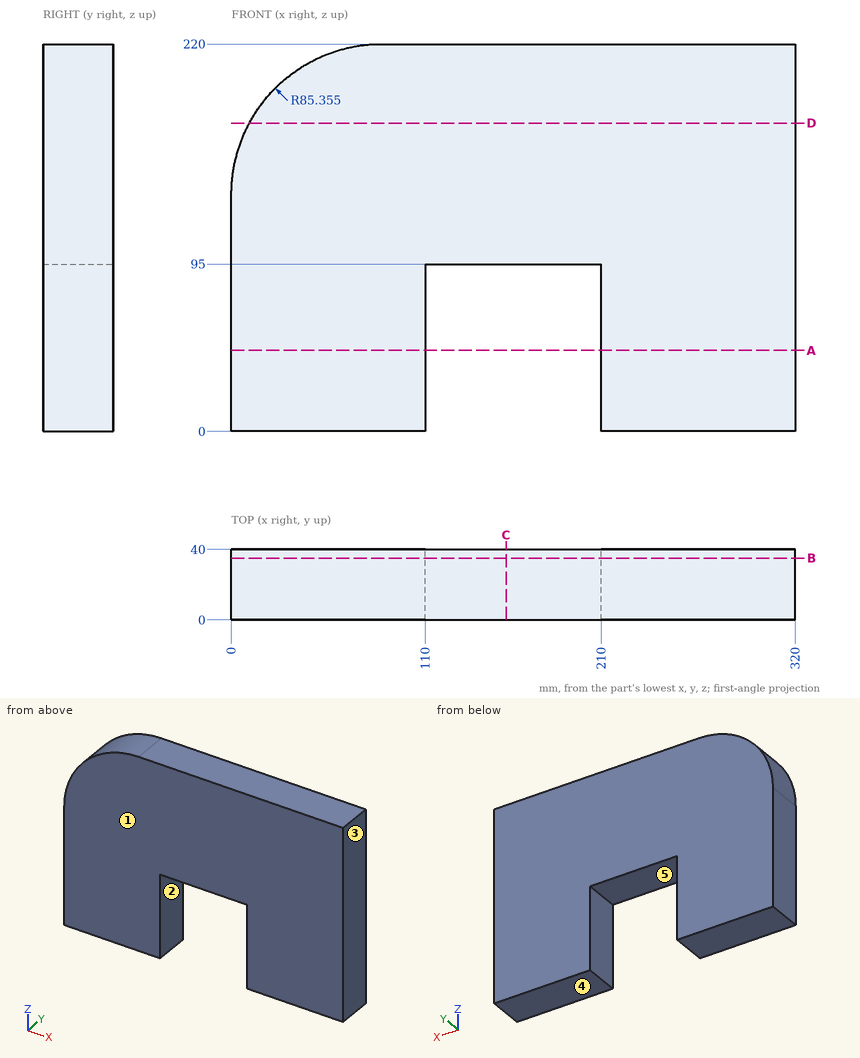
The drawing under review shows one solid part. Ordinate dimensions are in mm from its lowest x, y, z. A direction names the side the tool comes from. Round coordinates to 2 decimals unless told otherwise and drop trailing zeros. Order: outer loops, then holes, each group sorted by start corner. A loop starts at its lowest first (then second) coordinate and runs counter-clockwise, first axis right, second up. Notation, with made-up numbers: M -35,66 L -2,66 A28 cw -2,84 Z; hole C 51,75 d11. An arc over 180 degrees is marked long. Answer as CSV lines item,"result". Start each with the question number.
1) Wall thickness on line 1 along X through (y, z) = (7.5, 55.5); line 2 along Z through (x, y) = (160, 31.5); line 3 along Z through (x, y) = (77, 31): over which ranges is each line inside the solid? List them lowest first. Write a range as [from, to].
2) The part is to be moulded in two halves that separate along X. For the marked faces 3, 4 and 5, say which applies: +X half, -X half, draft (parallel to the pull), parting line (faces both ways), or undercut.
3) For pin 1 Ø10 at (y, z) = (20, 146.5) entering from -X, flat-tipped, find the tip position at first contact; note if it passes through.
4) Add section C-C (x = 156). Give the boundary of the cut face in (y, z).
5) Add section B-B (y = 35). Give the boundary of the cut face in (x, z) (1 decimal), then the cut area to 3 significant figures.
6) Add section D-D (z = 175). Give the boundary of the cut face in (x, y).
7) Tool access review of the marked faces 1 and 2: name each direction out of +Z, -Z, +X, -X, +Y, -Y from which nothing blocks a thin tool from reaching the whole face with its end or side.
8) Add section A-A (z = 46). Give the boundary of the cut face in (x, y), then the cut area to 3 significant figures.
Resolved:
1,line 1,"[0, 110], [210, 320]"
1,line 2,"[95, 220]"
1,line 3,"[0, 219.59]"
2,face 3,"+X half"
2,face 4,"draft"
2,face 5,"undercut"
3,pin 1,"x = 0.28"
4,outline,"M 0,95 L 40,95 L 40,220 L 0,220 Z"
5,outline,"M 0,0 L 110,0 L 110,95 L 210,95 L 210,0 L 320,0 L 320,220 L 85.4,220 A85.4 ccw 0,134.6 Z"
5,area,"59,300 mm^2"
6,outline,"M 10.14,0 L 320,0 L 320,40 L 10.14,40 Z"
7,face 1,"+Z, -Z, +X, -X, -Y"
7,face 2,"-Z, +Y, -Y"
8,outline,"M 0,0 L 110,0 L 110,40 L 0,40 Z; M 210,0 L 320,0 L 320,40 L 210,40 Z"
8,area,"8,800 mm^2"
